```python
from build123d import *

# Parameters (mm, degrees)
SKETCH_1_R          = 35
SKETCH_1_R_2        = 1.7
EXTRUDE_1_DEPTH     = 12
CUT_EXTRUDE_1_DEPTH = 6
SKETCH_4_R          = 14
CUT_EXTRUDE_3_DEPTH = 51.931326313
SKETCH_5_R          = 3.25
CUT_EXTRUDE_4_DEPTH = 8


with BuildPart() as part:
    # 草图1 → 凸台-拉伸1 (new body)
    with BuildSketch(Plane(origin=(0, 0, 0), x_dir=(1, 0, 0), z_dir=(0, 1, 0))):
        with Locations(Location((0, 0, 0), (0, 0, 270))):
            Circle(SKETCH_1_R)
        with Locations(Location((14.5, 25.11473671, 0), (0, 0, 270))):
            Circle(SKETCH_1_R_2, mode=Mode.SUBTRACT)
        with Locations(Location((14.5, -25.11473671, 0), (0, 0, 270))):
            Circle(SKETCH_1_R_2, mode=Mode.SUBTRACT)
        with Locations(Location((-29, 0, 0), (0, 0, 270))):
            Circle(SKETCH_1_R_2, mode=Mode.SUBTRACT)
    extrude(amount=EXTRUDE_1_DEPTH)

    # 草图2 → 切除-拉伸1 (cut)
    with BuildSketch(Plane(origin=(0, 12, 0), x_dir=(1, 0, 0), z_dir=(0, 1, 0))):
        with BuildLine():
            Line((35.785871092, 34.919499283), (-6.074470585, 10.348951981))
            ThreePointArc((-6.074470585, 10.348951981), (-11.954336377, -1.045868913), (-4.185109075, -11.246548894))
            Line((-4.185109075, -11.246548894), (41.305910715, -28.174842324))
            ThreePointArc((41.305910715, -28.174842324), (49.809734905, 4.357787137), (35.785871092, 34.919499283))
        make_face()
    extrude(amount=-CUT_EXTRUDE_1_DEPTH, mode=Mode.SUBTRACT)

    # 草图4 → 切除-拉伸3 (cut, through all)
    with BuildSketch(Plane.XZ):
        with Locations(Location((0, 0, 0), (0, 0, 270))):
            Circle(SKETCH_4_R)
    extrude(amount=-CUT_EXTRUDE_3_DEPTH, mode=Mode.SUBTRACT)

    # 草图5 → 切除-拉伸4 (cut)
    with BuildSketch(Plane(origin=(0, 12, 0), x_dir=(1, 0, 0), z_dir=(0, 1, 0))):
        with Locations(Location((14.5, 25.11473671, 0), (0, 0, 270))):
            Circle(SKETCH_5_R)
        with Locations(Location((14.5, -25.11473671, 0), (0, 0, 270))):
            Circle(SKETCH_5_R)
        with Locations(Location((-29, 0, 0), (0, 0, 270))):
            Circle(SKETCH_5_R)
    extrude(amount=-CUT_EXTRUDE_4_DEPTH, mode=Mode.SUBTRACT)


solid = part.part
```
Geometry check sheet. Reference: the model listing, model coordinates, mm. A direction names the side the tool comes from. Give positions to 0.01 mm unless a question says otherwise; leave off trailing zeros. Write each loop counter-clockwise with the first axis right and the second up, starting at its lowest first coordinate (ties: lowest second). Pieces come first, ordered by that corner, then holes.
1) Gauge pin test, flat ends, axial feed: pin 1 (3 mm diameter, centred on x = -30, z = 0, fed in from +Y); pin 2 (2 mm diameter, centred on x = 8, y = 5, fed in from +Z); pin 3 (3 mm diameter, centred on x = -20, y = 4, fed in from -Z); pin 4 (3 mm diameter, centred on x = -29, z = 0, fed in from +Y). Record the tip position at first contact, or that the pin passes through.
2) Material ranges on L1, parallel to X at y = 3.5, z = 0; L2, parallel to Z at x = 14.5, y = 1.1; L3, parallel to Z at x = 0, y = 3.25, recorded low to high.
3) Section check A-A, the plane y = 8.5. Record the boundary of the cut face in (x, z).
4) Section check C-C, the plane x = -29. Record the boundary of the cut face in (y, z), and give its area (3 significant figures).
5) Section check B-B, the plane z = 25.5. Record the boundary of the cut face in (x, y), and give its area (3 significant figures).
6) Access from +Z, -Z, +X, -X, +Y, -Y to the whole of each face (thin tool, end or side, straight path). Record for faces 4 (the flat face through (7.022, 9.042, -18.036)), 5 (the flat face through (13, 4, -24)), 6 (the cylindrical face through (13.849, 1.972, -23.544)).
7) Release check for a two-part mould opening along Z. For faces 1 (the flat face through (-17, 12, 0)), 2 (the cylindrical face through (-31.05, 5.92, 16.15)), 3 (the cylindrical face through (-32.173, 8.056, -0.705)) record: pulls with the +Z half, pulls with the -Z half, needs draft (parallel to the pull), parting line crosses it, or undercut.
8) Section check D-D, the plane z = 9. Record the boundary of the cut face in (x, y), and give its area (3 significant figures).
Computed:
1. pin 1: stops at y = 4
1. pin 2: stops at z = 34.29
1. pin 3: stops at z = -29.71
1. pin 4: passes through
2. L1: x = -35 to -30.7, -27.3 to -14, 14 to 35
2. L2: z = -31.86 to -26.81, -23.41 to 23.41, 26.81 to 31.86
2. L3: z = -35 to -14, 14 to 35
3. outline: (0.14, -14) arc R14 cw (long way) to (2.57, 13.76) - (26.63, 22.71) arc R35 ccw (long way) to (22.28, -26.99) - (17.64, -24.27) arc R3.25 cw (long way) to (13.71, -21.96) - close; hole circle Ø6.5 at (-29, 0); hole circle Ø6.5 at (14.5, 25.11)
4. outline: (0, -19.6) - (12, -19.6) - (12, -3.25) - (4, -3.25) - (4, -1.7) - (0, -1.7) - close; (0, 1.7) - (4, 1.7) - (4, 3.25) - (12, 3.25) - (12, 19.6) - (0, 19.6) - close
4. area: 405 mm2
5. outline: (-23.97, 0) - (12.84, 0) - (12.84, 4) - (11.27, 4) - (11.27, 12) - (-23.97, 12) - close; (16.16, 0) - (23.97, 0) - (23.97, 12) - (17.73, 12) - (17.73, 4) - (16.16, 4) - close
5. area: 510 mm2
6. face 4: +X, +Y
6. face 5: +Y
6. face 6: +Y, -Y
7. face 1: needs draft
7. face 2: parting line crosses it
7. face 3: undercut
8. outline: (-33.82, 0) - (-10.72, 0) - (-10.72, 12) - (-33.82, 12) - close; (10.72, 0) - (33.82, 0) - (33.82, 6) - (10.72, 6) - close
8. area: 416 mm2
